```python
from build123d import *

# Parameters (mm, degrees)
F1_DEPTH = 8.128
F2_W     = 7.37743
F2_H     = 9.382971
F2_W_2   = 7.954949
F2_H_2   = 10.831244
F3_DEPTH = 93.98


with BuildPart() as f1:
    # F0 (on Right) → F1 (new body)
    with BuildSketch(Plane.YZ):
        Polygon((76.068617, 0), (-76.462761, 0), (-76.265693, -31.333964), (76.068617, -31.333964), align=None)
    extrude(amount=F1_DEPTH)

    # F2 (on Top) → F3 (join)
    with BuildSketch(Plane.XY):
        with Locations((3.688715, -71.337815)):
            Rectangle(F2_W, F2_H)
        with Locations((3.977475, 70.281338)):
            Rectangle(F2_W_2, F2_H_2)
    extrude(amount=F3_DEPTH)


solid = f1.part
```
The listing builds one solid part. Answer for the finished solid, in the listing's coordinates (mm). A direction names the side the tool comes from. Round coordinates to 2 decimals unless told otherwise and drop trailing zeros. Loops run counter-clockwise (first coordinate to the right, second up) from the corner with the lowest first, then second, coordinate; pieces in that order, holes last.
Q1. Section B-B, the plane x = 5.75 is taken. Determine the outline of the cut face in (y, z).
Q2. Section C-C, the plane y = 58 is taken. Determine the outline of the cut face in (x, z), then the cut area to 3 significant figures.
Q3. Section A-A, the plane z = 4 is taken. Determine the outline of the cut face in (x, y).
Q4. Find the intervals of material crossed by line 1 (Y direction, x = 7, z = 80); line 2 (Z direction, x = 2.75, y = 48); line 3 (Y direction, x = 7.5, z = 31.5), in increasing order.
Q5. For a pull along Y with two mould halves and no side action, classify faces 1 (the face through (4, 1, 0)), 2 (the face through (4, -66.646, 46)), 3 (the face through (7.377, -71, 46)), 4 (the face through (4, -76.029, 46)) as released by +Y, released by -Y, zero draft, split by the parting line, or undercut.
Q6. Given pin 1 Ø10.5 at (y, z) = (-70, 41.5) entering from +X; pin 2 Ø1.5 at (x, z) = (4, 14.5) entering from +Y; pin 3 Ø1.5 at (y, z) = (-49.5, 1) entering from +X; pin 4 Ø12 at (y, z) = (71.5, 53) entering from +X, each flat-ended and moving along its own axis, determine where each tip first touches the part or whether it passes through.
Q7. Which of the six approach directions +Z, -Z, +X, -X, +Y, -Y give full straight-line access (tool end or side, diameter ignored) to faces 5 (the face through (4, 75.697, 46)), 6 (the face through (0, 70, 46)), 7 (the face through (4, 64.866, 46)), 8 (the face through (8.128, -1, -15)), 9 (the face through (7.955, 70, 46))?
Completed:
1. outline: (-76.46, 0) - (-76.27, -31.33) - (76.07, -31.33) - (76.07, 0) - (75.7, 0) - (75.7, 93.98) - (64.87, 93.98) - (64.87, 0) - (-66.65, 0) - (-66.65, 93.98) - (-76.03, 93.98) - (-76.03, 0) - close
2. outline: (0, -31.33) - (8.13, -31.33) - (8.13, 0) - (0, 0) - close
2. area: 255 mm2
3. outline: (0, -76.03) - (7.38, -76.03) - (7.38, -66.65) - (0, -66.65) - close; (0, 64.87) - (7.95, 64.87) - (7.95, 75.7) - (0, 75.7) - close
4. line 1: y = -76.03 to -66.65, 64.87 to 75.7
4. line 2: z = -31.33 to 0
4. line 3: y = 64.87 to 75.7
5. face 1: undercut
5. face 2: undercut
5. face 3: zero draft
5. face 4: released by -Y
6. pin 1: stops at x = 7.38
6. pin 2: stops at y = 75.7
6. pin 3: passes through
6. pin 4: stops at x = 7.95
7. face 5: +Z, +X, -X, +Y
7. face 6: +Z, -Z, -X, +Y, -Y
7. face 7: +Z, +X, -X
7. face 8: +Z, -Z, +X, +Y, -Y
7. face 9: +Z, +X, +Y, -Y
